from build123d import *

# Parameters (mm, degrees)
SKETCH1_W           = 30
SKETCH1_H           = 22
SKETCH1_R           = 5.15
BOSS_EXTRUDE1_DEPTH = 10
SKETCH2_R           = 2
CUT_EXTRUDE1_DEPTH  = 10
SKETCH7_R           = 1.2
CUT_EXTRUDE2_DEPTH  = 11


with BuildPart() as part:
    # Sketch1 → Boss-Extrude1 (new body)
    with BuildSketch(Plane.XY):
        Rectangle(SKETCH1_W, SKETCH1_H)
        Circle(SKETCH1_R, mode=Mode.SUBTRACT)
    extrude(amount=BOSS_EXTRUDE1_DEPTH)

    # Sketch2 → Cut-Extrude1 (cut)
    with BuildSketch(Plane.XZ.offset(11)):
        with Locations((-11, 5)):
            Circle(SKETCH2_R)
        with Locations((11, 5)):
            Circle(SKETCH2_R)
    extrude(amount=-CUT_EXTRUDE1_DEPTH, mode=Mode.SUBTRACT)

    # Sketch7 → Cut-Extrude2 (cut, through all)
    with BuildSketch(Plane.XY.offset(10)):
        with Locations((-8, 0)):
            Circle(SKETCH7_R)
        with Locations((8, 0)):
            Circle(SKETCH7_R)
    extrude(amount=-CUT_EXTRUDE2_DEPTH, mode=Mode.SUBTRACT)


solid = part.part
Could you check a few things on this model? Use its own coordinates, in mm. A direction names the side the tool comes from. Give positions to 0.01 mm unless a question says otherwise; leave off trailing zeros. Loops run counter-clockwise (first coordinate to the right, second up) from the corner with the lowest first, then second, coordinate; pieces in that order, holes last. Notation, with made-up numbers: (22, 15) -> (68, 15) arc R27 cw to (68, 42) -> close; hole circle Ø2 at (20.5, 21). An arc over 180 degrees is marked (long way). Answer as CSV lines item,"result". Start each with the question number.
(1) If we section it at D-D on y = -8.25: Write out the boundary of the cut face in (x, z).
(2) If we section it at B-B on x = 8: Write out the boundary of the cut face in (y, z), then the cut area to 3 significant figures.
(3) If we section it at C-C on z = 1.5: Write out the boundary of the cut face in (x, y), then the cut area to 3 significant figures.
(4) If we section it at A-A on y = 0: Write out the boundary of the cut face in (x, z), then the cut area to 3 significant figures.
(5) I'm going to push flat-ended pins straight in: pin 1 Ø4.5 at (x, z) = (-11, 4) entering from -Y; pin 2 Ø2 at (x, y) = (-8, 0) entering from -Z; pin 3 Ø1.2 at (x, z) = (10.5, 5) entering from -Y. Where does each tip first touch, or does it pass through?
(6) We'd pull the mould along X, two halves only. Please class faces 1 (the flat face through (-15, 0, 5)), 2 (the flat face through (3, -5, 0)), 3 (the cylindrical face through (-9.2, 0.05, 5.07)): released by +X, released by -X, zero draft, split by the parting line, or undercut.
(7) I need wall thicknesses on probe 1 along Y at (x, z) = (-8, 8.25); probe 2 along Z at (x, y) = (-11, -4); probe 3 along X at (y, z) = (0.5, 0.75). Which ranges of each line are inside material? Lowest first, please.
(8) Which directions (+Z, -Z, +X, -X, +Y, -Y) give clear straight access to the entire face, cutting with the end or side of a thin tool? Please do faces 4 (the cylindrical face through (4.91, 1.55, 4.93)), 5 (the flat face through (11, -1, 5)).
Computed:
1,outline,"(-15, 0) -> (15, 0) -> (15, 10) -> (-15, 10) -> close; hole circle Ø4 at (-11, 5); hole circle Ø4 at (11, 5)"
2,outline,"(-11, 0) -> (-1.2, 0) -> (-1.2, 10) -> (-11, 10) -> close; (1.2, 0) -> (11, 0) -> (11, 10) -> (1.2, 10) -> close"
2,area,"196 mm2"
3,outline,"(-15, -11) -> (15, -11) -> (15, 11) -> (-15, 11) -> close; hole circle Ø2.4 at (-8, 0); hole circle Ø10.3 at (0, 0); hole circle Ø2.4 at (8, 0)"
3,area,"568 mm2"
4,outline,"(-15, 0) -> (-9.2, 0) -> (-9.2, 10) -> (-15, 10) -> close; (-6.8, 0) -> (-5.15, 0) -> (-5.15, 10) -> (-6.8, 10) -> close; (5.15, 0) -> (6.8, 0) -> (6.8, 10) -> (5.15, 10) -> close; (9.2, 0) -> (15, 0) -> (15, 10) -> (9.2, 10) -> close"
4,area,"149 mm2"
5,pin 1,"stops at y = -11"
5,pin 2,"passes through"
5,pin 3,"stops at y = -1"
6,face 1,"released by -X"
6,face 2,"zero draft"
6,face 3,"undercut"
7,probe 1,"y = -11 to -1.2, 1.2 to 11"
7,probe 2,"z = 0 to 3, 7 to 10"
7,probe 3,"x = -15 to -9.09, -6.91 to -5.13, 5.13 to 6.91, 9.09 to 15"
8,face 4,"+Z, -Z"
8,face 5,"-Y"
